```python
from build123d import *

# Parameters (mm, degrees)
CUT_SWEEP1_PITCH = 4


with BuildPart() as part:
    # Sketch1 → Revolve1 (revolve)
    with BuildSketch(Plane.XY, mode=Mode.PRIVATE) as revolve1_sk:
        Polygon((7.495497647, 5), (7.495497647, 10), (-30.504502353, 10), (-30.504502353, 2.5), (-20.504502353, 2.5), (-20.504502353, 0), (-2.504502353, 0), (-2.504502353, 5), align=None)
    revolve(revolve1_sk.sketch.rotate(Axis((-30.504502353, 0, 0), (1, 0, 0)), 90), axis=Axis((-30.504502353, 0, 0), (1, 0, 0)))

    # Cut-Sweep1: arcs per turn and ends read off the stored shape
    # Cut-Sweep1: the profile of Sketch2 profile screwed along a right-hand helix through 3.25 turns, 12 arcs to a turn; built about Z, then put on its axis
    cut_sweep1_z = Axis((0, 0, 0), (0, 0, 1))
    cut_sweep1_corners = [(10.0003, 3.1417e-05, -7.495495647), (10.0003, 3.1417e-05, -10.495495647), (8, 2.5133e-05, -10.495495647), (8, 2.5133e-05, -7.495495647)]
    with BuildLine(mode=Mode.PRIVATE) as cut_sweep1_profile:
        Line(cut_sweep1_corners[0], cut_sweep1_corners[1])
        Line(cut_sweep1_corners[1], cut_sweep1_corners[2])
        Line(cut_sweep1_corners[2], cut_sweep1_corners[3])
        Line(cut_sweep1_corners[3], cut_sweep1_corners[0])
    cut_sweep1_cap = Face(cut_sweep1_profile.wire())
    cut_sweep1_turn_angles = [0, 15, 30, 45, 60, 75, 90, 105, 120, 135, 150, 165, 180, 195, 210, 225, 240, 255, 270, 285, 300, 315, 330, 345, 360]
    cut_sweep1_turn_weights = [1, 0.9659258262890683, 1, 0.9659258262890683, 1, 0.9659258262890683, 1, 0.9659258262890683, 1, 0.9659258262890683, 1, 0.9659258262890683, 1, 0.9659258262890683, 1, 0.9659258262890683, 1, 0.9659258262890683, 1, 0.9659258262890683, 1, 0.9659258262890683, 1, 0.9659258262890683, 1]
    cut_sweep1_turn_rails = [Edge.make_bspline([Vector(p[0], p[1], 0).rotate(cut_sweep1_z, cut_sweep1_turn_angles[k]) / cut_sweep1_turn_weights[k] + Vector(0, 0, p[2] + CUT_SWEEP1_PITCH * cut_sweep1_turn_angles[k] / 360) for k in range(25)], [0, 0, 0, 1, 1, 2, 2, 3, 3, 4, 4, 5, 5, 6, 6, 7, 7, 8, 8, 9, 9, 10, 10, 11, 11, 12, 12, 12], 2, cut_sweep1_turn_weights) for p in cut_sweep1_corners]
    cut_sweep1_turn_sides = [Face.make_surface_from_curves(cut_sweep1_turn_rails[p[0]], cut_sweep1_turn_rails[p[1]]) for p in [(0, 1), (1, 2), (2, 3), (3, 0)]]
    cut_sweep1_last_angles = [1080, 1095, 1110, 1125, 1140, 1155, 1170]
    cut_sweep1_last_weights = [1, 0.9659258262890683, 1, 0.9659258262890683, 1, 0.9659258262890646, 1]
    cut_sweep1_last_rails = [Edge.make_bspline([Vector(p[0], p[1], 0).rotate(cut_sweep1_z, cut_sweep1_last_angles[k]) / cut_sweep1_last_weights[k] + Vector(0, 0, p[2] + CUT_SWEEP1_PITCH * cut_sweep1_last_angles[k] / 360) for k in range(7)], [0, 0, 0, 1, 1, 2, 2, 3, 3, 3], 2, cut_sweep1_last_weights) for p in cut_sweep1_corners]
    cut_sweep1_last_sides = [Face.make_surface_from_curves(cut_sweep1_last_rails[p[0]], cut_sweep1_last_rails[p[1]]) for p in [(0, 1), (1, 2), (2, 3), (3, 0)]]
    cut_sweep1 = Plane(origin=(-14, 0, 0), x_dir=(0, 0, 1), z_dir=(-1, 0, 0)) * Solid(Shell([*[p.moved(Location((0, 0, CUT_SWEEP1_PITCH * i))) for i in range(3) for p in cut_sweep1_turn_sides], *cut_sweep1_last_sides, cut_sweep1_cap, cut_sweep1_cap.rotate(cut_sweep1_z, 1170).moved(Location((0, 0, CUT_SWEEP1_PITCH * 1170 / 360)))]))
    add(cut_sweep1, mode=Mode.SUBTRACT)


solid = part.part
```
Geometry: final body of the model. Coordinates: model frame, mm. A direction names the side the tool comes from. Round coordinates to 2 decimals unless told otherwise and drop trailing zeros. Write each loop counter-clockwise with the first axis right and the second up, starting at its lowest first coordinate (ties: lowest second). Pieces come first, ordered by that corner, then holes.
Item 1: Section query B-B (x = -3). Return loops of the section in (y, z), plus the area to 3 significant figures.
Item 2: Set-up query: faces 1 (the face through (-30.505, 2, 2)), 2 (the face through (3, 0, -5)), 3 (the face through (-25.4, -0.1, -2.5)). Return all of +Z, -Z, +X, -X, +Y, -Y with unobstructed straight access to the full face (end or side cutting, diameter ignored); none if empty.
Item 3: Pin query (flat end, axial travel): P1, Ø1, axis at x = -8.5, y = 5.5, coming from the -Z side; P2, Ø6, axis at x = -19.5, y = -2.5, coming from the -Z side; P3, Ø1.5, axis at x = -8, y = -2, coming from the +Z side; P4, Ø1.6, axis at x = -18, y = 9, coming from the +Z side. Return the tip coordinate at first contact, or that it passes through.
Item 4: Mould query, pull axis Y, two halves, no side actions, for faces 4 (the face through (7.495, -5, -2)), 5 (the face through (-20.505, 0, 0)). Classes: +Y half, -Y half, draft (parallel to the pull), parting line (faces both ways), or undercut.
Item 5: Section query A-A (x = 4.5). Return loops of the section in (y, z), plus the area to 3 significant figures.
Item 6: Material intervals for L1, parallel to Y at x = -26, z = 0; L2, parallel to X at y = -8.75, z = -1; L3, parallel to X at y = -8.5, z = 4.75, sorted ascending.
Completed:
1. outline: circle Ø20 at (0, 0)
1. area: 314 mm2
2. face 1: +Z, -Z, -X, +Y, -Y
2. face 2: +X
2. face 3: -X
3. P1: stops at z = -8.66
3. P2: stops at z = -10
3. P3: stops at z = 9.88
3. P4: stops at z = 0
4. face 4: draft
4. face 5: undercut
5. outline: circle Ø20 at (0, 0); hole circle Ø10 at (0, 0)
5. area: 236 mm2
6. L1: y = -10 to -2.5, 2.5 to 10
6. L2: x = -30.5 to -17.43, -14.43 to -13.43, -10.43 to -9.43, -6.43 to 7.5
6. L3: x = -30.5 to -17.83, -14.83 to -13.83, -10.83 to -9.83, -6.83 to 7.5
